Geometry check sheet. Reference: the model listing, model coordinates, mm. Coordinates: 2 decimals unless noted, no trailing zeros. Write each loop counter-clockwise with the first axis right and the second up, starting at its lowest first coordinate (ties: lowest second). Pieces come first, ordered by that corner, then holes.
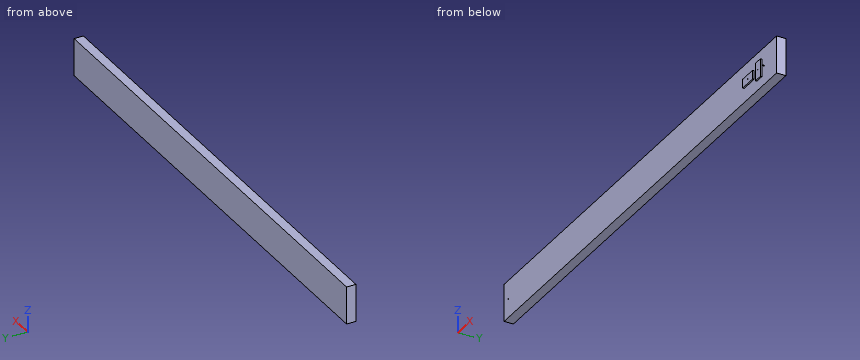
from build123d import *

# Parameters (mm, degrees)
F1_DEPTH = 6.3
F2_R     = 0.25
F3_DEPTH = 1
F4_R     = 0.25
F5_DEPTH = 1
F7_R     = 0.25
F8_DEPTH = 1
F6_R     = 0.25
F9_DEPTH = 1


with BuildPart() as f1:
    # F0 (on Front) → F1 (new body)
    with BuildSketch(Plane.XZ):
        Polygon((0, -12.69), (0, 0), (0, 12.69), (-317, 12.69), (-317, -12.69), align=None)
        Polygon((0, 12.69), (0, 0), (0, -12.69), (15, -12.69), (15, 12.69), align=None)
    extrude(amount=F1_DEPTH)

    # F2 (on face) → F3 (cut)
    with BuildSketch(Plane.XZ.offset(6.3)):
        with Locations((-312, 0)):
            Circle(F2_R)
    extrude(amount=-F3_DEPTH, mode=Mode.SUBTRACT)

    # F4 (on face) → F5 (cut)
    with BuildSketch(Plane.XZ.offset(6.3)):
        with Locations((-233, 0)):
            Circle(F4_R)
    extrude(amount=-F5_DEPTH, mode=Mode.SUBTRACT)

    # F7 (on face) → F8 (join)
    with BuildSketch(Plane.XZ.offset(6.3)):
        with BuildLine():
            ThreePointArc((0.25, 0), (0, 0.25), (-0.25, 0))
            ThreePointArc((-0.25, 0), (0, -0.25), (0.25, 0))
        make_face()
        with Locations((-6, 0)):
            Circle(F7_R)
        Polygon((-9, 6), (-9, 0), (-9, -6), (-3, -6), (-3, 0), (-3, 6), align=None)
        with Locations((-6, 0)):
            Circle(F7_R, mode=Mode.SUBTRACT)
    extrude(amount=F8_DEPTH)

    # F6 (on face) → F9 (join)
    with BuildSketch(Plane.XZ.offset(6.3)):
        with Locations((-18.5, 0)):
            Circle(F6_R)
        Polygon((-24.5, 3), (-24.5, 0), (-24.5, -3), (-18.5, -3), (-12.5, -3), (-12.5, 0), (-12.5, 3), (-18.5, 3), align=None)
        with Locations((-18.5, 0)):
            Circle(F6_R, mode=Mode.SUBTRACT)
    extrude(amount=F9_DEPTH)


solid = f1.part
1. Sectioned sample at B-B, the plane x = -122. Record the boundary of the cut face in (y, z), and give its area (3 significant figures).
Computed values:
outline: (-6.3, -12.69) - (0, -12.69) - (0, 12.69) - (-6.3, 12.69) - close
area: 160 mm2
2. Gauge pin test, flat ends, axial feed: pin 1 Ø5 at (x, z) = (-239, 7) entering from -Y; pin 2 Ø1.1 at (x, y) = (-20.5, -7) entering from -Z; pin 3 Ø0.8 at (y, z) = (-7, 2) entering from +X. Record the tip position at first contact, or that the pin passes through.
Computed values:
pin 1: stops at y = -6.3
pin 2: stops at z = -3
pin 3: stops at x = -3
3. Sectioned sample at A-A, the plane z = -9.75. Record the boundary of the cut face in (x, y).
Computed values:
outline: (-317, -6.3) - (15, -6.3) - (15, 0) - (-317, 0) - close
4. Thickness scan on line 1 along Z through (x, y) = (-233, -5.85); line 2 along Z through (x, y) = (-6, -6.6); line 3 along Y through (x, z) = (-147, -6). Record the ranges inside material, lowest first.
Computed values:
line 1: z = -12.69 to -0.25, 0.25 to 12.69
line 2: z = -6 to -0.25, 0.25 to 6
line 3: y = -6.3 to 0
